from build123d import *

# Parameters (mm, degrees)
SKETCH_1_R          = 12.5
EXTRUDE_1_DEPTH     = 4.8
SKETCH_2_R          = 15
EXTRUDE_2_DEPTH     = 8.7
SKETCH_3_R          = 14
EXTRUDE_3_DEPTH     = 7.6
SKETCH_6_R          = 5
CUT_EXTRUDE_1_DEPTH = 28.885659397


with BuildPart() as part:
    # 스케치1 → 보스-돌출1 (new body)
    with BuildSketch(Plane.XY):
        Circle(SKETCH_1_R)
    extrude(amount=EXTRUDE_1_DEPTH)

    # 스케치2 → 보스-돌출2 (add)
    with BuildSketch(Plane.XY.offset(4.8)):
        Circle(SKETCH_2_R)
    extrude(amount=EXTRUDE_2_DEPTH)

    # 스케치3 → 보스-돌출3 (add)
    with BuildSketch(Plane.XY.offset(13.5)):
        with Locations(Location((0, 0, 0), (0, 0, 180))):
            Circle(SKETCH_3_R)
    extrude(amount=EXTRUDE_3_DEPTH)

    # 스케치5 → 컷-회전1 (revolve, cut)
    with BuildSketch(Plane(origin=(0, 0, 0), x_dir=(1, 0, 0), z_dir=(0, 1, 0))):
        Polygon((0, -18.1), (5, -18.1), (9.8, -19.8), (12.4, -19.8), (12.4, -21.829479187), (0, -21.829479187), align=None)
    revolve(axis=Axis((0, 0, 21.829479187), (0, 0, -1)), mode=Mode.SUBTRACT)

    # 스케치6 → 컷-돌출1 (cut, through all)
    with BuildSketch(Plane.XY.offset(18.1)):
        Circle(SKETCH_6_R)
    extrude(amount=-CUT_EXTRUDE_1_DEPTH, mode=Mode.SUBTRACT)


solid = part.part
Verification items for the finished model (mm, model axes). A direction names the side the tool comes from. Give positions to 0.01 mm unless a question says otherwise; leave off trailing zeros. Order: outer loops, then holes, each group sorted by start corner. A loop starts at its lowest first (then second) coordinate and runs counter-clockwise, first axis right, second up. Notation, with made-up numbers: M 48,-11.75 L 79,-11.75 A20 ccw 79,19.25 Z; hole C -6,-8.75 d4. An arc over 180 degrees is marked long. Use one line per item in the form item = value. Start each with the question number.
Q1. Section check C-C (z = 7.75). Enter the section's corners in (x, y).
Q2. Mould release check, pull along X, two halves, no side actions. Record for faces 4 (the flat face through (-1, -10, 19.8)), 5 (the flat face through (-3.4, 12.3, 4.8)), 6 (the cylindrical face through (-14.985, 0.66, 9.089)): +X half, -X half, draft (parallel to the pull), parting line (faces both ways), or undercut.
Q3. Section check D-D (z = 2.75). Enter the section's corners in (x, y).
Q4. Scan lines: line 1 along Y through (x, z) = (0, 8); line 2 along Y through (x, z) = (0, 20.15); line 3 along Z through (x, y) = (3.5, -12.75). Record each from-to range of solid material in increasing order. Write a range as [from, to].
Q5. Access from +Z, -Z, +X, -X, +Y, -Y to the whole of each face (thin tool, end or side, straight path). Record for faces 1 (the cylindrical face through (-12.932, 5.362, 17.247)), 2 (the cylindrical face through (11.923, 3.755, 2.366)), 3 (the flat face through (2.1, 12.4, 21.1)).
Q6. Section check A-A (y = 0). Enter the section's corners in (x, z).
Q7. Go/stop test with flat-tipped pins: pin 1 Ø4 at (y, z) = (8, 12) entering from -X; pin 2 Ø8 at (x, z) = (7.5, 18) entering from -Y; pin 3 Ø7.5 at (x, y) = (-4, 1.5) entering from +Z. Record where each tip stops, or that it passes through.
Evaluation:
q1.outline = C 0,0 d30; hole C 0,0 d10
q2.face_4 = undercut
q2.face_5 = draft
q2.face_6 = parting line
q3.outline = C 0,0 d25; hole C 0,0 d10
q4.line_1 = [-15, -5], [5, 15]
q4.line_2 = [-14, -12.4], [12.4, 14]
q4.line_3 = [4.8, 21.1]
q5.face_1 = +Z
q5.face_2 = -Z
q5.face_3 = +Z, +X, -X, +Y, -Y
q6.outline = M -15,4.8 L -12.5,4.8 L -12.5,0 L -5,0 L -5,18.1 L -9.8,19.8 L -12.4,19.8 L -12.4,21.1 L -14,21.1 L -14,13.5 L -15,13.5 Z; M 5,0 L 12.5,0 L 12.5,4.8 L 15,4.8 L 15,13.5 L 14,13.5 L 14,21.1 L 12.4,21.1 L 12.4,19.8 L 9.8,19.8 L 5,18.1 Z
q7.pin_1 = -13.75
q7.pin_2 = -13.56
q7.pin_3 = 19.17
